Here's the drawing with two shaded views (mm, measured from the low corner). I have some questions. A direction names the side the tool comes from. Round coordinates to 2 decimals unless told otherwise and drop trailing zeros. Write each loop counter-clockwise with the first axis right and the second up, starting at its lowest first coordinate (ties: lowest second). Pieces come first, ordered by that corner, then holes. Notation, with made-up numbers: M 64,67.25 L 116,67.25 A22 ccw 116,75.25 Z; hole C 8.5,39 d4. An arc over 180 degrees is marked long. Write item = value, one per line. Start each with the question number.
(1) Will these pins go through, and if not, where does the flat tip stop? pin 1 Ø12 at (x, z) = (18.5, 24) entering from -Y; pin 2 Ø3 at (x, z) = (19.5, 7) entering from -Y.
(2) If we mould it in two halves opening along Z, with no side actions, what happens to the marked faces 1, 2 and 3? For each: released by +Z, released by -Z, zero draft, split by the parting line, or undercut.
(3) On a 3-axis mill with a long thin cutter (end or side, diameter ignored), from which of +Z, -Z, +X, -X, +Y, -Y can I reach the whole of each face in a straight line? I mean the marked faces 4 and 5. Say none if no direction works.
(4) I want a section at D-D (z = 19). List the corners of the cut face in (x, y) for me, and give its area (3 significant figures).
(5) I want a section at A-A (y = 13). List the corners of the cut face in (x, z) for me.
(6) I need wall thicknesses on line 1 along Y through (x, z) = (10.5, 25); line 2 along Z through (x, y) = (30.5, 27.5); line 3 along Y through (x, z) = (17, 6.5). Which ranges of each line are inside material? Lowest first, please.
(7) I want a section at C-C (x = 36). List the corners of the cut face in (y, z) for me (1 decimal).
(8) I want a section at B-B (x = 19). List the corners of the cut face in (y, z) for me.
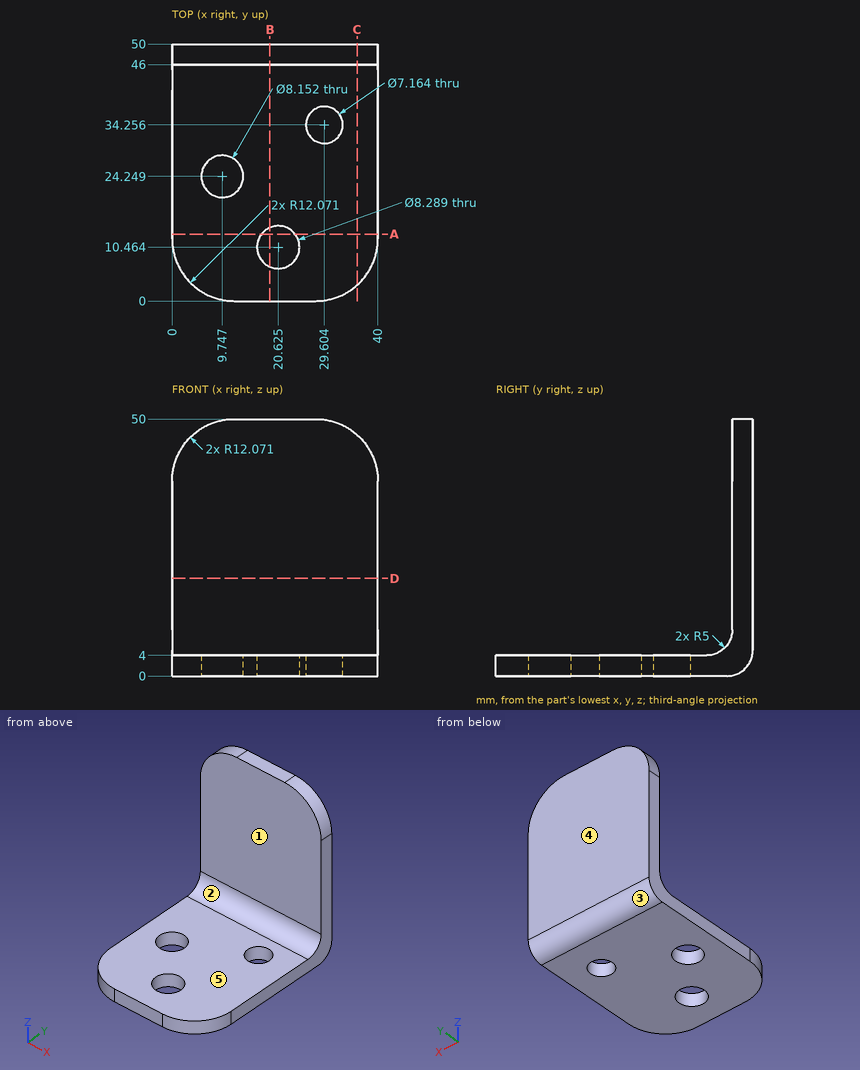
Returned:
q1.pin_1 = 46
q1.pin_2 = 44.57
q2.face_1 = zero draft
q2.face_2 = released by +Z
q2.face_3 = released by -Z
q3.face_4 = +Z, -Z, +X, -X, +Y
q3.face_5 = +Z, +X, -X, -Y
q4.outline = M 0,46 L 40,46 L 40,50 L 0,50 Z
q4.area = 160 mm²
q5.outline = M 0,0 L 17.35,0 L 17.35,4 L 0,4 Z; M 23.9,0 L 40,0 L 40,4 L 23.9,4 Z
q6.line_1 = 46 to 50
q6.line_2 = 0 to 4
q6.line_3 = 45.33 to 50
q7.outline = M 3.1,0 L 45,0 A5 ccw 50,5 L 50,46.9 L 46,46.9 L 46,9 A5 cw 41,4 L 3.1,4 Z
q8.outline = M 0,0 L 6.65,0 L 6.65,4 L 0,4 Z; M 14.28,0 L 45,0 A5 ccw 50,5 L 50,50 L 46,50 L 46,9 A5 cw 41,4 L 14.28,4 Z
